Build history of the part. All positions in model axes, mm. A direction names the side the tool comes from. Round coordinates to 2 decimals unless told otherwise and drop trailing zeros. Write each loop counter-clockwise with the first axis right and the second up, starting at its lowest first coordinate (ties: lowest second). Pieces come first, ordered by that corner, then holes.
Item 1: Mould opens along Y. For faces 3 (the flat face through (0, 7, 18.05)), 4 (the flat face through (0, -17.5, 9)), 5 (the flat face through (0, -15.525, 10)) say: +Y half, -Y half, draft (parallel to the pull), parting line (faces both ways), or undercut.
Item 2: 3-axis set-ups, long thin cutter, end or side, ignore diameter. For faces 1 (the flat face through (0, -13, 18.05)), 2 (the flat face through (0, -7.916, 10)): which of +Z, -Z, +X, -X, +Y, -Y reach the whole face in a straight line?
Item 3: Band-saw the part on B-B, the plane y = -2. Write the cut outline in (x, z), then the cut area to 3 significant figures.
Item 4: Wall check: probe 1 along Z at (x, y) = (6, -2.5). Give the ranges that are in metal, low to high.
Item 5: Band-saw the part on A-A, the plane z = 12.75. Count the separate pieces of the cut face and the enclosed holes in it, then the cut area to 3 significant figures.
Item 6: Drop flat-ended pins along their axis: pin 1 Ø2 at (y, z) = (-8.5, 10) entering from -X; pin 2 Ø0.5 at (x, y) = (0.5, -15) entering from +Z. Give the stop position or say it passes through.
```python
from build123d import *

# Parameters (mm, degrees)
BOX_W                = 35
BOX_H                = 35
BOX_DEPTH            = 1.5
BOX017_W             = 1.9755
BOX017_H             = 35
BOX017_DEPTH         = 16.5
BOX018_W             = 1.9755
BOX018_H             = 35
BOX018_DEPTH         = 16.5
BOX019_W             = 1.9755
BOX019_H             = 35
BOX019_DEPTH         = 16.5
BOX020_W             = 1.9755
BOX020_H             = 35
BOX020_DEPTH         = 16.5
BOX021_W             = 1.9755
BOX021_H             = 35
BOX021_DEPTH         = 16.5
BOX022_W             = 1.9755
BOX022_H             = 35
BOX022_DEPTH         = 16.5
BOX023_W             = 1.9755
BOX023_H             = 35
BOX023_DEPTH         = 16.5
BOX024_W             = 1.9755
BOX024_H             = 35
BOX024_DEPTH         = 16.5
BOX025_W             = 1.9755
BOX025_H             = 35
BOX025_DEPTH         = 16.5
BOX026_W             = 1.9755
BOX026_H             = 35
BOX026_DEPTH         = 16.5
BODY_PLACEMENT_ANGLE = 90


with BuildPart() as part:
    # Box → Box (join)
    with BuildSketch(Plane(origin=(-17.5, -17.5, 0), x_dir=(1, 0, 0), z_dir=(0, 0, 1))):
        with Locations((17.5, 17.5)):
            Rectangle(BOX_W, BOX_H)
    extrude(amount=BOX_DEPTH)

    # Box017 → Box017 (join)
    with BuildSketch(Plane(origin=(15.5245, -17.5, 1.5), x_dir=(1, 0, 0), z_dir=(0, 0, 1))):
        with Locations((0.98775, 17.5)):
            Rectangle(BOX017_W, BOX017_H)
    extrude(amount=BOX017_DEPTH)

    # Box018 → Box018 (join)
    with BuildSketch(Plane(origin=(12.481022, -17.5, 1.5), x_dir=(1, 0, 0), z_dir=(0, 0, 1))):
        with Locations((0.98775, 17.5)):
            Rectangle(BOX018_W, BOX018_H)
    extrude(amount=BOX018_DEPTH)

    # Box019 → Box019 (join)
    with BuildSketch(Plane(origin=(9.437544, -17.5, 1.5), x_dir=(1, 0, 0), z_dir=(0, 0, 1))):
        with Locations((0.98775, 17.5)):
            Rectangle(BOX019_W, BOX019_H)
    extrude(amount=BOX019_DEPTH)

    # Box020 → Box020 (join)
    with BuildSketch(Plane(origin=(6.394066, -17.5, 1.5), x_dir=(1, 0, 0), z_dir=(0, 0, 1))):
        with Locations((0.98775, 17.5)):
            Rectangle(BOX020_W, BOX020_H)
    extrude(amount=BOX020_DEPTH)

    # Box021 → Box021 (join)
    with BuildSketch(Plane(origin=(3.350588, -17.5, 1.5), x_dir=(1, 0, 0), z_dir=(0, 0, 1))):
        with Locations((0.98775, 17.5)):
            Rectangle(BOX021_W, BOX021_H)
    extrude(amount=BOX021_DEPTH)

    # Box022 → Box022 (join)
    with BuildSketch(Plane(origin=(-4.872327, -17.5, 1.5), x_dir=(1, 0, 0), z_dir=(0, 0, 1))):
        with Locations((0.98775, 17.5)):
            Rectangle(BOX022_W, BOX022_H)
    extrude(amount=BOX022_DEPTH)

    # Box023 → Box023 (join)
    with BuildSketch(Plane(origin=(-7.915805, -17.5, 1.5), x_dir=(1, 0, 0), z_dir=(0, 0, 1))):
        with Locations((0.98775, 17.5)):
            Rectangle(BOX023_W, BOX023_H)
    extrude(amount=BOX023_DEPTH)

    # Box024 → Box024 (join)
    with BuildSketch(Plane(origin=(-10.959283, -17.5, 1.5), x_dir=(1, 0, 0), z_dir=(0, 0, 1))):
        with Locations((0.98775, 17.5)):
            Rectangle(BOX024_W, BOX024_H)
    extrude(amount=BOX024_DEPTH)

    # Box025 → Box025 (join)
    with BuildSketch(Plane(origin=(-14.002761, -17.5, 1.5), x_dir=(1, 0, 0), z_dir=(0, 0, 1))):
        with Locations((0.98775, 17.5)):
            Rectangle(BOX025_W, BOX025_H)
    extrude(amount=BOX025_DEPTH)

    # Box026 → Box026 (join)
    with BuildSketch(Plane(origin=(-17.5, -17.5, 1.5), x_dir=(1, 0, 0), z_dir=(0, 0, 1))):
        with Locations((0.98775, 17.5)):
            Rectangle(BOX026_W, BOX026_H)
    extrude(amount=BOX026_DEPTH)


with BuildPart() as part_1:
    # Body placement: moved
    add(part.part.moved(Location((0, 0, 0.05))).rotate(Axis((0, 0, 0.05), (0, 0, 1)), BODY_PLACEMENT_ANGLE))


solid = part_1.part
```
Results:
1. face 3: draft
1. face 4: -Y half
1. face 5: undercut
2. face 1: +Z, +X, -X, +Y, -Y
2. face 2: +Z, +X, -X
3. outline: (-17.5, 0.05) - (17.5, 0.05) - (17.5, 1.55) - (-17.5, 1.55) - close
3. area: 52.5 mm2
4. probe 1: z = 0.05 to 1.55
5. separate pieces: 10
5. enclosed holes: 0
5. area: 691 mm2
6. pin 1: stops at x = -17.5
6. pin 2: stops at z = 1.55
